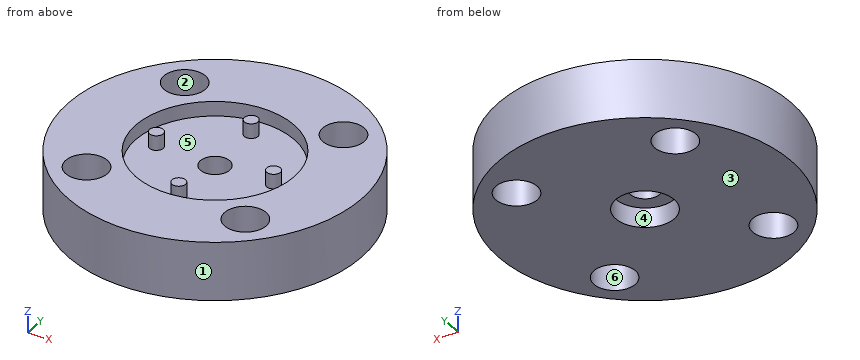
```python
from build123d import *

# Parameters (mm, degrees)
SKETCH1_R           = 15
SKETCH1_R_2         = 2.125
SKETCH1_R_3         = 1.5
BOSS_EXTRUDE1_DEPTH = 6
SKETCH2_R           = 8.1
SKETCH2_R_2         = 0.7
CUT_EXTRUDE1_DEPTH  = 1.5
SKETCH3_R           = 3
CUT_EXTRUDE2_DEPTH  = 2


with BuildPart() as part:
    # Sketch1 → Boss-Extrude1 (new body)
    with BuildSketch(Plane.XY):
        Circle(SKETCH1_R)
        with Locations((8.136527837, 8.126925295)):
            Circle(SKETCH1_R_2, mode=Mode.SUBTRACT)
        with Locations((8.136527837, -8.136530672)):
            Circle(SKETCH1_R_2, mode=Mode.SUBTRACT)
        with Locations((-8.12692813, -8.136530672)):
            Circle(SKETCH1_R_2, mode=Mode.SUBTRACT)
        with Locations((-8.12692813, 8.126925295)):
            Circle(SKETCH1_R_2, mode=Mode.SUBTRACT)
        Circle(SKETCH1_R_3, mode=Mode.SUBTRACT)
    extrude(amount=BOSS_EXTRUDE1_DEPTH)

    # Sketch2 → Cut-Extrude1 (cut)
    with BuildSketch(Plane.XY.offset(6)):
        Circle(SKETCH2_R)
        with Locations((0, 6)):
            Circle(SKETCH2_R_2, mode=Mode.SUBTRACT)
        with Locations((6, 0)):
            Circle(SKETCH2_R_2, mode=Mode.SUBTRACT)
        with Locations((0, -6)):
            Circle(SKETCH2_R_2, mode=Mode.SUBTRACT)
        with Locations((-6, 0)):
            Circle(SKETCH2_R_2, mode=Mode.SUBTRACT)
    extrude(amount=-CUT_EXTRUDE1_DEPTH, mode=Mode.SUBTRACT)

    # Sketch3 → Cut-Extrude2 (cut)
    with BuildSketch(Plane(origin=(0, 0, 0), x_dir=(-1, 0, 0), z_dir=(0, 0, -1))):
        Circle(SKETCH3_R)
    extrude(amount=-CUT_EXTRUDE2_DEPTH, mode=Mode.SUBTRACT)


solid = part.part
```
Design review of the part built by this model. Coordinates are the model's own, in mm. Face numbers are marked on the shaded views. A direction names the side the tool comes from. Give positions to 0.01 mm unless a question says otherwise; leave off trailing zeros. Order: outer loops, then holes, each group sorted by start corner. A loop starts at its lowest first (then second) coordinate and runs counter-clockwise, first axis right, second up. Notation, with made-up numbers: (20, 62) - (28, 62) arc R27 cw to (28, 81) - close; hole circle Ø5 at (84.5, 81.5). An arc over 180 degrees is marked (long way). Use a Markdown table: item, result. Add a question column.
(1) Wall thickness on probe 1 along Y at (x, z) = (0, 5.3); probe 2 along Y at (x, z) = (0, 0.5); probe 3 along X at (y, z) = (-10, 3.85): over which ranges is each line inside the solid? List them lowest first. Write a range as [from, to].
(2) Add section A-A on x = 0. Give the boundary of the cut face in (y, z), then the cut area to 3 significant figures.
(3) Add section B-B on z = 5.4. Give the number of separate pieces and of enclosed holes in the cut face, then the cut area to 3 significant figures.
(4) Add section C-C on y = -4.25. Give the boundary of the cut face in (x, z), then the cut area to 3 significant figures.
(5) Mouldability with a two-part tool opening along Y and no side actions: class the marked faces 1, 2 and 3 as +Y half, -Y half, draft (parallel to the pull), parting line (faces both ways), or undercut.
(6) Add section D-D on z = 3.65. Give the boundary of the cut face in (x, y) (3 decimals), then the cut area to 3 significant figures.
(7) Machinability: for the marked faces 4, 5 and 6, which of the approach directions +Z, -Z, +X, -X, +Y, -Y give a long, thin tool a straight path to every point of the face, cutting with its end or side? Answer none if there is none.
(8) Clearance check with flat-ended pins moving along their axes: P1, Ø1, axis at x = -6, z = 1.5, coming from the -Y side; P2, Ø5, axis at x = 2.5, y = 0, coming from the +Z side; P3, Ø1, axis at x = -10, z = 2.5, coming from the -Y side; P4, Ø2.5, axis at x = 8.14, y = 8.13, coming from the -Z side. State where each tip first meets the part, or that it passes through.
Report:
| question | item | result |
|---|---|---|
| 1 | probe 1 | y = [-15, -8.1], [-6.7, -5.3], [5.3, 6.7], [8.1, 15] |
| 1 | probe 2 | y = [-15, -3], [3, 15] |
| 1 | probe 3 | x = [-11.18, -9.15], [-7.11, 7.12], [9.16, 11.18] |
| 2 | outline | (-15, 0) - (-3, 0) - (-3, 2) - (-1.5, 2) - (-1.5, 4.5) - (-5.3, 4.5) - (-5.3, 6) - (-6.7, 6) - (-6.7, 4.5) - (-8.1, 4.5) - (-8.1, 6) - (-15, 6) - close; (1.5, 2) - (3, 2) - (3, 0) - (15, 0) - (15, 6) - (8.1, 6) - (8.1, 4.5) - (6.7, 4.5) - (6.7, 6) - (5.3, 6) - (5.3, 4.5) - (1.5, 4.5) - close |
| 2 | area | 140 mm² |
| 3 | separate pieces | 5 |
| 3 | enclosed holes | 5 |
| 3 | area | 450 mm² |
| 4 | outline | (-14.39, 0) - (14.39, 0) - (14.39, 6) - (6.9, 6) - (6.9, 4.5) - (-6.9, 4.5) - (-6.9, 6) - (-14.39, 6) - close |
| 4 | area | 152 mm² |
| 5 | face 1 | parting line |
| 5 | face 2 | undercut |
| 5 | face 3 | draft |
| 6 | outline | circle Ø30 at (0, 0); hole circle Ø4.25 at (-8.127, -8.137); hole circle Ø4.25 at (-8.127, 8.127); hole circle Ø3 at (0, 0); hole circle Ø4.25 at (8.137, -8.137); hole circle Ø4.25 at (8.137, 8.127) |
| 6 | area | 643 mm² |
| 7 | face 4 | -Z |
| 7 | face 5 | +Z |
| 7 | face 6 | +Z, -Z |
| 8 | P1 | stops at y = -13.96 |
| 8 | P2 | stops at z = 4.5 |
| 8 | P3 | stops at y = -11.61 |
| 8 | P4 | passes through |
